The listing builds one solid part. Answer for the finished solid, in the listing's coordinates (mm). Round coordinates to 2 decimals unless told otherwise and drop trailing zeros. Write each loop counter-clockwise with the first axis right and the second up, starting at its lowest first coordinate (ties: lowest second). Pieces come first, ordered by that corner, then holes. Notation, with made-up numbers: (60, 23.25) - (106, 23.25) arc R35 ccw to (106, 57.25) - close; hole circle Ø6 at (26, 77). An arc over 180 degrees is marked (long way). Answer in a Markdown table with one row per item.
Autodesk Inventor part; units mm, degrees
ref_plane "YZ Plane" through (0, 0, 0) normal (1, 0, 0) x (0, 1, 0)
ref_plane "XZ Plane" through (0, 0, 0) normal (0, 1, 0) x (-1, 0, 0)
ref_plane "XY Plane" through (0, 0, 0) normal (0, 0, 1) x (1, 0, 0)
sketch "Sketch1" plane through (0, 0, 0) normal (0, 1, 0) x (-1, 0, 0)
  line L0 (0, 0) -> (-152.4, 0)
  line L1 (-152.4, 0) -> (-152.4, -76.2)
  line L2 (-152.4, -76.2) -> (0, -76.2)
  line L3 (0, -76.2) -> (0, 0)
  circle A0 centre (-25.4, -38.1) radius 4.7625
  circle A1 centre (-127, -38.1) radius 4.7625
  dimension "d0" = 152.4
  dimension "d1" = 76.2
  dimension "d3" = 9.525
  dimension "d7" = 9.525
extrude "Plate1" add sketch "Sketch1" along normal blind 3.048
equation "\"d8\" = Thickness"
equation "\"BendRadius\" = Thickness"
equation "\"BendReliefWidth\" = Thickness"
equation "\"BendReliefDepth\" = 0.5 * Thickness"
equation "\"CornerReliefSize\" = 4 * Thickness"
equation "\"MinimumRemnant\" = 2 * Thickness"
equation "\"TransitionRadius\" = BendRadius"
equation "\"JacobiRadiusSize\" = BendRadius"
equation "\"GapSize\" = Thickness"
properties part number "6x3"
(1) For a pull along X with two mould halves and no side action, classify faces 1 (the flat face through (152.4, 2, -38)), 2 (the flat face through (0, 2, -39)), 3 (the cylindrical face through (131.758, 1.503, -38.309)), 4 (the flat face through (77, 3.048, -38)) as pulls with the +X half, pulls with the -X half, needs draft (parallel to the pull), parting line crosses it, or undercut.
Checked values:
| item | result |
|---|---|
| face 1 | pulls with the +X half |
| face 2 | pulls with the -X half |
| face 3 | undercut |
| face 4 | needs draft |
(2) A flat-ended cylindrical pin translates along its axis: pin 1 (7.5 mm diameter, centred on x = 127, z = -38.1, fed in from +Y). Find the tip coordinate at first contact, or state that the pin passes through.
Checked values:
| item | result |
|---|---|
| pin 1 | passes through |
(3) Section A-A (z = -38.1) is taken. Give the vertices of the cut face in (x, y).
Checked values:
| item | result |
|---|---|
| outline | (0, 0) - (20.64, 0) - (20.64, 3.05) - (0, 3.05) - close; (30.16, 0) - (122.24, 0) - (122.24, 3.05) - (30.16, 3.05) - close; (131.76, 0) - (152.4, 0) - (152.4, 3.05) - (131.76, 3.05) - close |
(4) Section B-B (x = 25.4) is taken. Give the vertices of the cut face in (y, z), and give its area (3 significant figures).
Checked values:
| item | result |
|---|---|
| outline | (0, -76.2) - (3.05, -76.2) - (3.05, -42.86) - (0, -42.86) - close; (0, -33.34) - (3.05, -33.34) - (3.05, 0) - (0, 0) - close |
| area | 203 mm2 |
(5) Find the intervals of material crossed by line 1 (Z direction, x = 127, y = 0.75); line 2 (Z direction, x = 123, y = 2.5), in increasing order.
Checked values:
| item | result |
|---|---|
| line 1 | z = -76.2 to -42.86, -33.34 to 0 |
| line 2 | z = -76.2 to -40.68, -35.52 to 0 |
